Verification items for the finished model (mm, model axes). Face numbers are marked on the shaded views. Give positions to 0.01 mm unless a question says otherwise; leave off trailing zeros. Loops run counter-clockwise (first coordinate to the right, second up) from the corner with the lowest first, then second, coordinate; pieces in that order, holes last. Notation, with made-up numbers: M -23,-31 L 35,-31 A27 ccw 35,2 Z; hole C 1,46 d6. An arc over 180 degrees is marked long. Use a Markdown table: item, result.
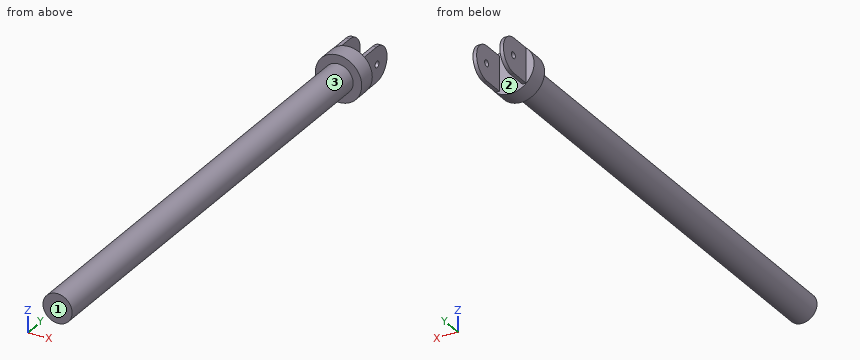
from build123d import *

# Parameters (mm, degrees)
SKETCH1_R           = 25.4
BOSS_EXTRUDE1_DEPTH = 19.05
SKETCH2_R           = 3.5
BOSS_EXTRUDE2_DEPTH = 4
SKETCH3_R           = 16
BOSS_EXTRUDE3_DEPTH = 508


with BuildPart() as part:
    # Sketch1 → Boss-Extrude1 (new body)
    with BuildSketch(Plane(origin=(0, 0, 0), x_dir=(1, 0, 0), z_dir=(0, 1, 0))):
        Circle(SKETCH1_R)
    extrude(amount=BOSS_EXTRUDE1_DEPTH)

    # Sketch2 → Boss-Extrude2 (add)
    with BuildSketch(Plane(origin=(12.7, 0, 0), x_dir=(0, 0, -1), z_dir=(1, 0, 0))):
        with BuildLine():
            Line((-19, 19.05), (19, 19.05))
            Line((19, 19.05), (19, 41.05))
            ThreePointArc((19, 41.05), (0, 60.05), (-19, 41.05))
            Line((-19, 41.05), (-19, 19.05))
        make_face()
        with Locations((0, 42.05)):
            Circle(SKETCH2_R, mode=Mode.SUBTRACT)
    boss_extrude2 = extrude(amount=BOSS_EXTRUDE2_DEPTH)

    # Mirror1: Boss-Extrude2 across plane
    add(boss_extrude2.mirror(Plane(origin=(0, 0, 0), x_dir=(0, 0, 1), z_dir=(1, 0, 0))))

    # Sketch3 → Boss-Extrude3 (add)
    with BuildSketch(Plane.XZ):
        Circle(SKETCH3_R)
    extrude(amount=BOSS_EXTRUDE3_DEPTH)


solid = part.part
(1) Draft check along X on the marked faces 1, 2 and 3. Enter one of: +X half, -X half, draft (parallel to the pull), parting line (faces both ways), or undercut.
Results below:
| item | result |
|---|---|
| face 1 | draft |
| face 2 | undercut |
| face 3 | parting line |
(2) Cross-section at B-B on y = -390.5. Record the cut outline in (x, z).
Results below:
| item | result |
|---|---|
| outline | C 0,0 d32 |
(3) Cross-section at A-A on x = 0. Record the cut outline in (y, z), then the cut area to 3 significant figures.
Results below:
| item | result |
|---|---|
| outline | M -508,-16 L 0,-16 L 0,-25.4 L 19.05,-25.4 L 19.05,25.4 L 0,25.4 L 0,16 L -508,16 Z |
| area | 17,200 mm^2 |
(4) Material ranges on line 1 (Y direction, x = -14.4, z = 0); line 2 (X direction, y = 19.5, z = -6); line 3 (Y direction, x = 2, z = 6.5), recorded low to high.
Results below:
| item | result |
|---|---|
| line 1 | -508 to 38.55, 45.55 to 60.05 |
| line 2 | -16.7 to -12.7, 12.7 to 16.7 |
| line 3 | -508 to 19.05 |
(5) Gauge pin test, flat ends, axial feed: P1, Ø4, axis at x = -13, y = -338, coming from the -Z side; P2, Ø3, axis at x = 18.5, z = 9, coming from the -Y side; P3, Ø11.5, axis at y = 43.5, z = 5, coming from the +X side. Record the tip position at first contact, or that the pin passes through.
Results below:
| item | result |
|---|---|
| P1 | z = -11.62 |
| P2 | y = 0 |
| P3 | x = 16.7 |
